Verification items for this drawing (mm, ordinates from the low corner). Give positions to 0.01 mm unless a question says otherwise; leave off trailing zeros. Loops run counter-clockwise (first coordinate to the right, second up) from the corner with the lowest first, then second, coordinate; pieces in that order, holes last. Notation, with made-up numbers: (16, 61.5) -> (41, 61.5) arc R26 ccw to (41, 96.5) -> close; hole circle Ø3 at (38, -7). An arc over 180 degrees is marked (long way). Answer in a Markdown table with one row per item. Add a question column.
Q1. Section check A-A on y = 25.8. Enter the section's corners in (x, z).
Q2. Material ranges on probe 1 along X at (y, z) = (25.8, 8); probe 2 along X at (y, z) = (37, 18), recorded low to high.
Q3. Section check C-C on z = 35.5. Enter the section's corners in (x, y).
Q4. Section check B-B on x = 39.5. Enter the section's corners in (y, z), and give its area (3 significant figures).
Q5. Gauge pin test, flat ends, axial feed: P1, Ø3, axis at y = 6, z = 16, coming from the -X side; P2, Ø10, axis at x = 16, z = 7.5, coming from the +Y side; P3, Ø2, axis at y = 43.5, z = 23, coming from the +X side; P4, Ø10, axis at x = 21, z = 12, coming from the +Y side. Record the tip position at first contact, or that the pin passes through.
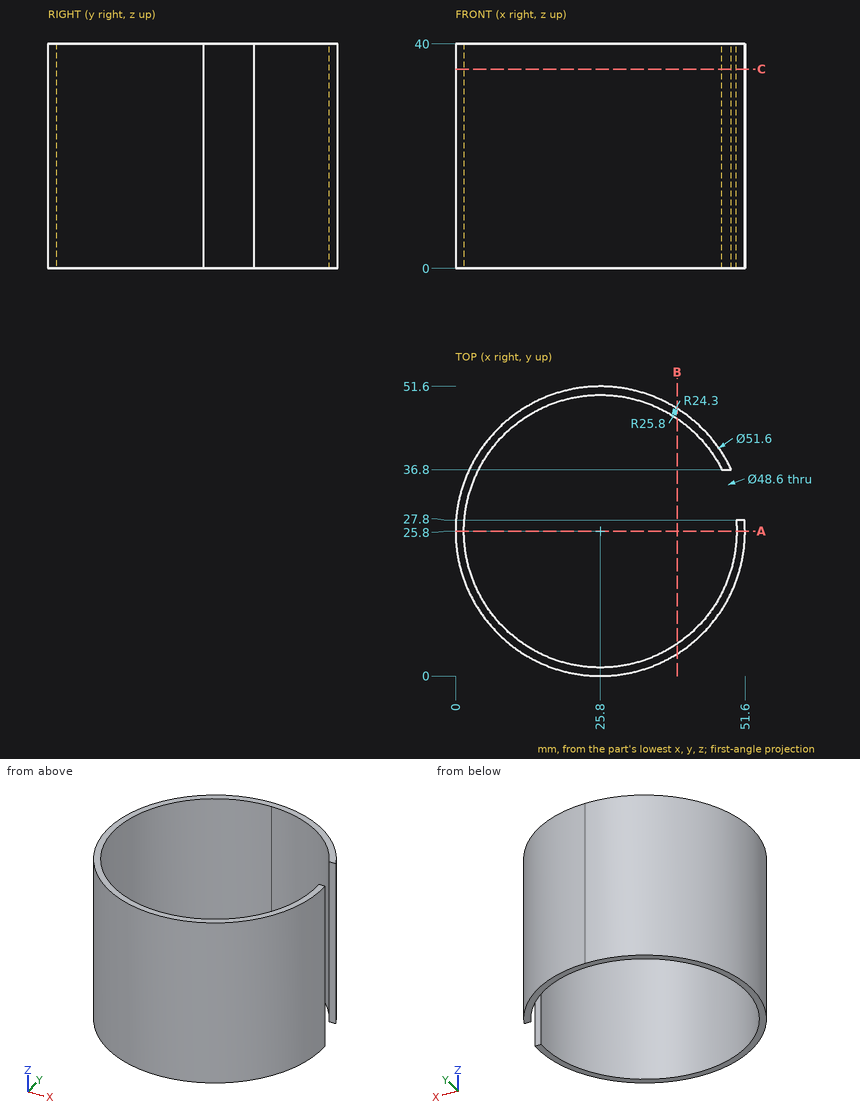
Taken from the geometry:
| question | item | result |
|---|---|---|
| 1 | outline | (0, 0) -> (1.5, 0) -> (1.5, 40) -> (0, 40) -> close; (50.1, 0) -> (51.6, 0) -> (51.6, 40) -> (50.1, 40) -> close |
| 2 | probe 1 | x = 0 to 1.5, 50.1 to 51.6 |
| 2 | probe 2 | x = 2.56 to 4.23, 47.37 to 49.04 |
| 3 | outline | (47.47, 36.8) -> (49.14, 36.8) arc R25.8 ccw (long way) to (51.52, 27.8) -> (50.02, 27.8) arc R24.3 cw (long way) to start |
| 4 | outline | (3.94, 0) -> (5.73, 0) -> (5.73, 40) -> (3.94, 40) -> close; (45.87, 0) -> (47.66, 0) -> (47.66, 40) -> (45.87, 40) -> close |
| 4 | area | 143 mm² |
| 5 | P1 | stops at x = 7.61 |
| 5 | P2 | stops at y = 51.15 |
| 5 | P3 | stops at x = 45.47 |
| 5 | P4 | stops at y = 51.6 |
